Autodesk Inventor part; units mm, degrees
ref_plane "YZ Plane" through (0, 0, 0) normal (1, 0, 0) x (0, 1, 0)
ref_plane "XZ Plane" through (0, 0, 0) normal (0, 1, 0) x (-1, 0, 0)
ref_plane "XY Plane" through (0, 0, 0) normal (0, 0, 1) x (1, 0, 0)
sketch "Sketch1" plane through (0, 0, 0) normal (0, 1, 0) x (-1, 0, 0)
  line L0 (43, 16) -> (43, -16)
  line L1 (43, -16) -> (0, -16)
  line L2 (0, -16) -> (0, 0)
  line L3 (0, 0) -> (23, 0)
  line L4 (39, 16) -> (39, 16)
  line L5 (39, 16) -> (43, 16)
  arc A0 (23, 0) -> (39, 16) centre (23, 16) ccw
  dimension "d0" = 16
  dimension "d1" = 32
  dimension "d2" = 4
  dimension "d3" = 16
  dimension "d4" = 43
extrude "Extrusion1" add sketch "Sketch1" along normal blind 16
fillet "Fillet1" radius 2 6 edges at (-34.3137, 16, 4.6863) (-11.5, 16, 0) (-21.5, 16, -16) (-21.5, 0, -16) (-34.3137, 0, 4.6863) (-11.5, 0, 0)
ref_plane "Work Plane1" through (-39, 0, 16) normal (-1, 0, 0) x (0, 0, 1)
sketch "Sketch2" plane through (-39, 0, 16) normal (-1, 0, 0) x (0, 0, 1)
  line L0 (-16, 14) -> (0, 14)
  line L1 (0, 2) -> (-16, 2)
  line L2 (-14, 14) -> (0, 14)
  line L3 (0, 14) -> (0, 2)
  line L4 (0, 2) -> (-14, 2)
  line L5 (-16, 4) -> (-16, 12)
  arc A0 (-14, 14) -> (-16, 12) centre (-14, 12) ccw
  arc A1 (-16, 4) -> (-14, 2) centre (-14, 4) ccw
  point P0 (-16, 0)
  dimension "d9" = 2
  dimension "d10" = 16
extrude "Extrusion2" cut sketch "Sketch2" against normal blind 16
sketch "Sketch3" plane through (-39, 0, 16) normal (1, 0, 0) x (0, 0, -1)
  line L0 (0, 0) -> (18, 0)
  line L1 (18, 16) -> (0, 16)
  line L2 (0, 2) -> (0, 14)
  point P0 (16, 0)
  point P1 (8, 8)
  dimension "d13" = 16
  dimension "d14" = 8
  dimension "d15" = 8
hole "Hole1" at (-39, 8, 8) direction (-1, 0, 0) diameter 6.756 depth 8.8
sketch "Sketch4" plane through (0, 0, -2) normal (1, 0, 0) x (0, 0, -1)
  line L0 (0, 16) -> (12, 16)
  line L1 (14, 2) -> (14, 14)
  line L2 (0.475, 14) -> (2.525, 14) construction
  line L3 (0.475, 12.975) -> (2.525, 12.975)
  line L4 (2.525, 15.025) -> (0.475, 15.025)
  arc A0 (0.475, 15.025) -> (0.475, 12.975) centre (0.475, 14) ccw
  arc A1 (2.525, 12.975) -> (2.525, 15.025) centre (2.525, 14) ccw
  line L5 (9.475, 2) -> (11.525, 2) construction
  line L6 (9.475, 0.975) -> (11.525, 0.975)
  line L7 (11.525, 3.025) -> (9.475, 3.025)
  arc A2 (9.475, 3.025) -> (9.475, 0.975) centre (9.475, 2) ccw
  arc A3 (11.525, 0.975) -> (11.525, 3.025) centre (11.525, 2) ccw
  point P0 (-2, 0)
  point P1 (6, 8)
  point P2 (1.5, 14)
  point P3 (10.5, 2)
  dimension "d23" = 8
  dimension "d24" = 8
  dimension "d25" = 9
  dimension "d26" = 4.5
  dimension "d27" = 2.05
  dimension "d28" = 2.05
  dimension "d29" = 2.05
  dimension "d30" = 2.05
  dimension "d31" = 12
  dimension "d32" = 6
extrude "Extrusion3" add sketch "Sketch4" along normal blind 1.5
hole "Hole2" at (0, 8, -8) direction (-1, 0, 0) diameter 4.978 depth 19.05
equation "\"d1\" = 2 * d0"
equation "\"d28\" = d27"
equation "\"d29\" = d28"
equation "\"d30\" = d29"
properties part number "vive_mount"
Input: part model. Units: mm. Frame: model coordinates. A direction names the side the tool comes from. Round coordinates to 2 decimals unless told otherwise and drop trailing zeros. Write each loop counter-clockwise with the first axis right and the second up, starting at its lowest first coordinate (ties: lowest second). Pieces come first, ordered by that corner, then holes. Notation, with made-up numbers: (-24, -21.75) - (8, -21.75) arc R22 cw to (8, -10.75) - close; hole circle Ø10 at (37.25, 38). An arc over 180 degrees is marked (long way). Write item = value, one per line.
(1) Contact query for flat-ended pins moving along their axis: pin 1 Ø5 at (y, z) = (9, 10) entering from +X; pin 2 Ø1.5 at (y, z) = (10, -2.5) entering from +X; pin 3 Ø0.8 at (x, z) = (0.5, -3.5) entering from +Y (3 decimals). Output: stop coordinate, or through.
Geometry check:
pin_1 = -39
pin_2 = 0
pin_3 = 15.025
(2) Access query for faces 4 (the cylindrical face through (0.74, 2.02, -14.55)), 5 (the cylindrical face through (-41.028, 10.997, 6.441)), 6 (the flat face through (1, 0.975, -12)), 7 (the flat face through (1, 3.025, -13)), 8 (the flat face through (-37, 2, 5)). Directions: +Z, -Z, +X, -X, +Y, -Y. A direction counts if a zero-diameter tool reaches every point of the face in a straight line with its end or side. Return the directions, or none.
Geometry check:
face_4 = -Z, +X
face_5 = +X, -X
face_6 = +Z, -Z, +X, -Y
face_7 = +Z, -Z, +X, +Y
face_8 = +Z, +X
(3) Section query A-A on y = 8. Output: boundary loops of the cut face in (x, z).
Geometry check:
outline = (-43, -16) - (0, -16) - (0, -10.49) - (-19.05, -10.49) - (-19.05, -5.51) - (0, -5.51) - (0, 0) - (-39, 0) - (-39, 4.62) - (-43, 4.62) - close; (-43, 11.38) - (-39, 11.38) - (-39, 16) - (-43, 16) - close
(4) Pull-direction query (Z, two-part tool) for faces 1 (the cylindrical face through (-11.66, 15.4, -0.57)), 2 (the flat face through (1.5, 14, -3)), 3 (the flat face through (-19.05, 8, -8)); classes: +Z half, -Z half, draft (parallel to the pull), parting line (faces both ways), or undercut.
Geometry check:
face_1 = +Z half
face_2 = draft
face_3 = undercut
(5) Section query C-C on x = -14. Output: boundary loops of the cut face in (y, z).
Geometry check:
outline = (0, -14) arc R2 ccw to (2, -16) - (14, -16) arc R2 ccw to (16, -14) - (16, -2) arc R2 ccw to (14, 0) - (2, 0) arc R2 ccw to (0, -2) - close; hole circle Ø4.98 at (8, -8)
(6) Section query B-B on z = -12. Output: boundary loops of the cut face in (x, y) (3 decimals).
Geometry check:
outline = (-43, 0) - (0, 0) - (0, 0.975) - (1.5, 0.975) - (1.5, 3.025) - (0, 3.025) - (0, 16) - (-43, 16) - close
(7) Section query D-D on x = -21. Output: boundary loops of the cut face in (y, z), then the cut area to 3 significant figures.
Geometry check:
outline = (0, -14) arc R2 ccw to (2, -16) - (14, -16) arc R2 ccw to (16, -14) - (16, -2) arc R2 ccw to (14, 0) - (2, 0) arc R2 ccw to (0, -2) - close
area = 253 mm^2
(8) Material intervals for probe 1 along Y at (x, z) = (-9, -8); probe 2 along Z at (x, y) = (-40.6, 8); probe 3 along Z at (x, y) = (-9.75, 8), sorted ascending.
Geometry check:
probe_1 = 0 to 5.51, 10.49 to 16
probe_2 = -16 to 4.62, 11.38 to 16
probe_3 = -16 to -10.49, -5.51 to 0
